The listing builds one solid part. Answer for the finished solid, in the listing's coordinates (mm). A direction names the side the tool comes from. Round coordinates to 2 decimals unless told otherwise and drop trailing zeros. Loops run counter-clockwise (first coordinate to the right, second up) from the corner with the lowest first, then second, coordinate; pieces in that order, holes last. Notation, with made-up numbers: (63, 79.5) -> (101, 79.5) arc R16 cw to (101, 98.5) -> close; hole circle Ø1 at (-24.5, -11.5). An arc over 180 degrees is marked (long way). One line per question, with ' | ' between items.
from build123d import *

# Parameters (mm, degrees)
DODANIE_WYCI_GNI_CIE1_DEPTH = 15
ZAOKR_GLENIE1_R             = 5
ZAOKR_GLENIE2_R             = 1
SZKIC3_R                    = 11
DODANIE_WYCI_GNI_CIE2_DEPTH = 6


with BuildPart() as part:
    # Szkic1 → Dodanie-wyci_gni_cie1 (new body)
    with BuildSketch(Plane.XY):
        Polygon((14.43375673, -25), (28.867513459, 0), (14.43375673, 25), (-14.43375673, 25), (-28.867513459, 0), (-14.43375673, -25), align=None)
    extrude(amount=DODANIE_WYCI_GNI_CIE1_DEPTH)

    # Zaokr_glenie1
    zaokr_glenie1_edges = [part.edges().sort_by_distance(p)[0] for p in [
        (21.650635095, 12.5, 15),
        (0, 25, 15),
        (-21.650635095, 12.5, 15),
        (-21.650635095, -12.5, 15),
        (0, -25, 15),
        (21.650635095, -12.5, 15),
    ]]
    fillet(zaokr_glenie1_edges, radius=ZAOKR_GLENIE1_R)

    # Zaokr_glenie2
    zaokr_glenie2_edges = [part.edges().sort_by_distance(p)[0] for p in [
        (-14.43375673, 25, 5),
        (14.43375673, 25, 5),
        (-28.867513459, 0, 5),
        (-14.43375673, -25, 5),
        (14.43375673, -25, 5),
        (28.867513459, 0, 5),
        (13.514121691, -23.407145389, 13.65942076),
        (-13.514121691, -23.407145389, 13.65942076),
        (27.028243383, 0, 13.65942076),
        (-27.02824329, 0, 13.659420835),
        (13.514121691, 23.407145389, 13.65942076),
        (-13.514121691, 23.407145389, 13.65942076),
    ]]
    fillet(zaokr_glenie2_edges, radius=ZAOKR_GLENIE2_R)

    # Szkic3 → Dodanie-wyci_gni_cie2 (add)
    with BuildSketch(Plane(origin=(0, 0, 0), x_dir=(-1, 0, 0), z_dir=(0, 0, -1))):
        with Locations(Location((0, 0, 0), (0, 0, 180))):
            Circle(SZKIC3_R)
        Polygon((4.618802154, -8), (9.237604307, 0), (4.618802154, 8), (-4.618802154, 8), (-9.237604307, 0), (-4.618802154, -8), align=None, mode=Mode.SUBTRACT)
    extrude(amount=DODANIE_WYCI_GNI_CIE2_DEPTH)


solid = part.part
Q1. For a pull along Y with two mould halves and no side action, classify faces 1 (the face through (0, 8, -3)), 2 (the face through (0, -25, 5)), 3 (the face through (6, 6, -6)) as pulls with the +Y half, pulls with the -Y half, needs draft (parallel to the pull), parting line crosses it, or undercut.
Numbers:
face 1: undercut | face 2: pulls with the -Y half | face 3: needs draft
Q2. A cutting plane is placed at C-C on x = 0. Give the vertices of the cut face in (y, z).
Numbers:
outline: (-25, 0) -> (-11, 0) -> (-11, -6) -> (-8, -6) -> (-8, 0) -> (8, 0) -> (8, -6) -> (11, -6) -> (11, 0) -> (25, 0) -> (25, 10) arc R5 ccw to (20, 15) -> (-20, 15) arc R5 ccw to (-25, 10) -> close
Q3. Given pin 1 Ø3 at (x, y) = (20, -19) entering from -Z; pin 2 Ø5 at (x, z) = (-1, -3) entering from -Y; pin 3 Ø5 at (x, z) = (11.5, -3.5) entering from +Y; pin 4 Ø5 at (y, z) = (-14, 5) entering from +X, each flat-ended and moving along its own axis, determine where each tip first touches the part or whether it passes through.
Numbers:
pin 1: through | pin 2: y = -11 | pin 3: y = 6.32 | pin 4: x = 22.23
Q4. A cutting plane is placed at B-B on z = 4.5. Give the vertices of the cut face in (x, y), plus the area to 3 significant figures.
Numbers:
outline: (-28.58, -0.5) -> (-14.72, -24.5) arc R1 ccw to (-13.86, -25) -> (13.86, -25) arc R1 ccw to (14.72, -24.5) -> (28.58, -0.5) arc R1 ccw to (28.58, 0.5) -> (14.72, 24.5) arc R1 ccw to (13.86, 25) -> (-13.86, 25) arc R1 ccw to (-14.72, 24.5) -> (-28.58, 0.5) arc R1 ccw to start | area: 2,160 mm^2
Q5. A cutting plane is placed at A-A on z = -3.25. Give the vertices of the cut face in (x, y).
Numbers:
outline: circle Ø22 at (0, 0); hole (-9.24, 0) -> (-4.62, -8) -> (4.62, -8) -> (9.24, 0) -> (4.62, 8) -> (-4.62, 8) -> close
Q6. Find the intervals of material crossed by line 1 (Z direction, x = 0, y = 19); line 2 (Y direction, x = -6, z = -2.75); line 3 (X direction, y = 20.5, z = 0.5), in increasing order. Write a range as from..to.
Numbers:
line 1: 0..15 | line 2: -9.22..-5.61, 5.61..9.22 | line 3: -17.03..17.03
Q7. A cutting plane is placed at D-D on x = -10. Give the vertices of the cut face in (y, z).
Numbers:
outline: (-25, 0) -> (-4.58, 0) -> (-4.58, -6) -> (4.58, -6) -> (4.58, 0) -> (25, 0) -> (25, 10) arc R5 ccw to (20, 15) -> (-20, 15) arc R5 ccw to (-25, 10) -> close
Q8. For faces 4 (the face through (20.51, -11.62, 13.5)), 5 (the face through (6.961, -3.944, -2.958)), determine the directions among +Z, -Z, +X, -X, +Y, -Y from which every point of the face is accessible in a straight line to the end or side of a thin tool.
Numbers:
face 4: +Z, +X, -Y | face 5: -Z
